Autodesk Inventor part; units mm, degrees
ref_plane "YZ Plane" through (0, 0, 0) normal (1, 0, 0) x (0, 1, 0)
ref_plane "XZ Plane" through (0, 0, 0) normal (0, 1, 0) x (-1, 0, 0)
ref_plane "XY Plane" through (0, 0, 0) normal (0, 0, 1) x (1, 0, 0)
sketch "Sketch1" plane through (0, 0, 0) normal (0, 1, 0) x (-1, 0, 0)
  line L0 (0, -34.641) -> (30, 17.3205) construction
  line L1 (30, 17.3205) -> (-30, 17.3205) construction
  line L2 (-30, 17.3205) -> (0, -34.641) construction
  circle A0 centre (0, 0) radius 34.641 construction
  circle A1 centre (0, -34.641) radius 10
  circle A2 centre (-30, 17.3205) radius 10
  circle A3 centre (30, 17.3205) radius 10
  circle A4 centre (0, 0) radius 20
  line L3 (55, -55) -> (-55, -55)
  line L4 (-55, -55) -> (-55, 55)
  line L5 (-55, 55) -> (55, 55)
  line L6 (55, 55) -> (55, -55)
  circle A5 centre (0, 0) radius 45 construction
  point P0 (0, -55)
  point P1 (55, 0)
  dimension "d0" = 60
  dimension "d1" = 20
  dimension "d2" = 40
  dimension "d3" = 90
  dimension "d4" = 55
extrude "Extrusion1" add sketch "Sketch1" against normal blind 110
sketch "Sketch2" plane through (0, 0, 0) normal (0, 1, 0) x (1, 0, 0)
  circle A0 centre (0, 0) radius 20
  circle A1 centre (-30, -17.3205) radius 10
  circle A2 centre (30, -17.3205) radius 10
  circle A3 centre (0, 34.641) radius 10
  line L0 (-55, 55) -> (55, 55)
  line L1 (-55, -55) -> (-55, 55)
  line L2 (55, -55) -> (-55, -55)
  line L3 (55, 55) -> (55, -55)
  circle A4 centre (0, 34.641) radius 6.25
  circle A5 centre (-30, 17.3205) radius 6.25
  circle A6 centre (-30, -17.3205) radius 6.25
  circle A7 centre (0, -34.641) radius 6.25
  circle A8 centre (30, -17.3205) radius 6.25
  circle A9 centre (30, 17.3205) radius 6.25
  arc A10 (-35.4127, 20.4455) -> (-35.4127, -20.4455) centre (0, 0) ccw
  arc A11 (-24.5873, 14.1955) -> (-24.5873, -14.1955) centre (0, 0) ccw
  arc A12 (0, -40.891) -> (35.4127, -20.4455) centre (0, 0) ccw
  arc A13 (35.4127, 20.4455) -> (0, 40.891) centre (0, 0) ccw
  arc A14 (0, -28.391) -> (24.5873, -14.1955) centre (0, 0) ccw
  arc A15 (24.5873, 14.1955) -> (0, 28.391) centre (0, 0) ccw
  dimension "d7" = 12.5
  dimension "d10" = 360
extrude "Extrusion2" cut sketch "Sketch2" against normal through all contours A11 A6 A10 A1 | A1 A10 A5 A11 | A5 | A14 A8 A12 A2 | A2 A12 A7 A14 | A7 | A3 A15 A4 A13 | A3 A13 A9 A15 | A9 picked at (-34.5635, -9.9186) picked at (25.4365, -24.7224) picked at (8.6846, 33.9839)
sketch "Sketch3" plane through (0, -110, 0) normal (0, -1, 0) x (1, 0, 0)
  line L0 (-55, -55) -> (55, -55)
  line L1 (55, -55) -> (55, 55)
  line L2 (55, 55) -> (-55, 55)
  line L3 (-55, 55) -> (-55, -55)
  arc A0 (7.0121, -27.5115) -> (24.5873, -14.1955) centre (0, 0) ccw
  arc A1 (35.4127, -20.4455) -> (24.5873, -14.1955) centre (30, -17.3205) ccw
  arc A2 (8.4355, -40.0115) -> (35.4127, -20.4455) centre (0, 0) ccw
  arc A3 (7.0121, -27.5115) -> (8.4355, -40.0115) centre (0, -34.641) ccw
  arc A4 (20.3196, 19.8284) -> (0, 28.391) centre (0, 0) ccw
  arc A5 (0, 40.891) -> (0, 28.391) centre (0, 34.641) ccw
  arc A6 (30.4332, 27.3111) -> (0, 40.891) centre (0, 0) ccw
  arc A7 (20.3196, 19.8284) -> (30.4332, 27.3111) centre (30, 17.3205) ccw
  arc A8 (-27.3317, 7.6831) -> (-24.5873, -14.1955) centre (0, 0) ccw
  arc A9 (-35.4127, -20.4455) -> (-24.5873, -14.1955) centre (-30, -17.3205) ccw
  arc A10 (-38.8687, 12.7003) -> (-35.4127, -20.4455) centre (0, 0) ccw
  arc A11 (-27.3317, 7.6831) -> (-38.8687, 12.7003) centre (-30, 17.3205) ccw
  circle A12 centre (0, 0) radius 20
  line L4 (-50, 50) -> (50, 50)
  line L5 (50, 50) -> (50, -50)
  line L6 (50, -50) -> (-50, -50)
  line L7 (-50, -50) -> (-50, 50)
  dimension "d14" = 5
extrude "Extrusion3" cut sketch "Sketch3" against normal blind 100 contours A0 A1 A2 A3 | A4 A5 A6 A7 | A8 A9 A10 A11 | A12 | L4 L5 L6 L7
sketch "Sketch5" plane through (55, 0, -55) normal (0, 0, -1) x (-1, 0, 0)
  circle A0 centre (55, -60) radius 10
  line L0 (110, -110) -> (0, -110)
  line L1 (110, 0) -> (0, 0)
  point P0 (55, 0)
  point P1 (55, -110)
  dimension "d17" = 60
  dimension "d20" = 20
extrude "Extrusion4" cut sketch "Sketch5" against normal through all
sketch "Sketch6" plane through (55, 0, 55) normal (1, 0, 0) x (0, 0, -1)
  circle A0 centre (55, -60) radius 10
  line L0 (110, -110) -> (0, -110)
  line L1 (110, 0) -> (0, 0)
  point P0 (55, 0)
  point P1 (55, -110)
  dimension "d21" = 20
  dimension "d22" = 60
extrude "Extrusion5" cut sketch "Sketch6" against normal up to next
sketch "Sketch7" plane through (-50, -110, 50) normal (1, 0, 0) x (0, 0, -1)
  circle A0 centre (90, 15) radius 5
  line L0 (105, 110) -> (105, 0)
  line L1 (-5, 0) -> (105, 0)
  point P0 (50, 110)
  dimension "d25" = 10
  dimension "d26" = 15
  dimension "d27" = 15
extrude "Extrusion6" cut sketch "Sketch7" against normal through all
properties part number "Case1" material "Steel, Mild, Welded"
CAD build for the part. Positions are in the model's coordinates, mm. A direction names the side the tool comes from. Round coordinates to 2 decimals unless told otherwise and drop trailing zeros. Order: outer loops, then holes, each group sorted by start corner. A loop starts at its lowest first (then second) coordinate and runs counter-clockwise, first axis right, second up. Notation, with made-up numbers: (48.5, -40) -> (102.5, -40) arc R34 cw to (102.5, -3) -> close; hole circle Ø1 at (1, 7.25). An arc over 180 degrees is marked (long way). Write item = value, one per line. Start each with the question number.
(1) Pull direction Y, two halves, no side cores. Call faces 1 (the cylindrical face through (-52, -98, -36)), 2 (the flat face through (-1, -72, 50)), 3 (the flat face through (4, -110, -53)): released by +Y, released by -Y, zero draft, split by the parting line, or undercut.
(2) Cut at B-B, the plane y = -23. List the corners of the cut face in (x, z).
(3) Which spindle directions (+Z, -Z, +X, -X, +Y, -Y) get a long thin tool onto all of the face, cutting with end or side? Do faces 4 (the cylindrical face through (52.54, -69.76, 2.17)), 5 (the flat face through (1, -42, 55)), 6 (the flat face through (-50, -61, -1)), 7 (the cylindrical face through (-6.25, -4.93, 34.5)). Say none if no direction does.
(4) Probe line 1 (Z direction, x = -8.5, y = -38); line 2 (Z direction, x = -30, y = -4.75). List the from-to ranges inside material, lowest first. Write a range as [from, to].
(5) Cut at A-A, the plane x = -12. List the corners of the cut face in (y, z), then the cut area to 3 significant figures.
(6) Pin check, flat tip, straight feed: P1, Ø1, axis at x = 40.5, z = -1, coming from the -Y side. Stop position of the tip, or through.
(7) Cut at D-D, the plane y = -60. List the corners of the cut face in (x, z), then the cut area to 3 significant figures.
(8) Cut at C-C, the plane z = 0. List the corners of the cut face in (x, y).
Model answer:
q1.face_1 = undercut
q1.face_2 = zero draft
q1.face_3 = released by -Y
q2.outline = (-55, -55) -> (55, -55) -> (55, 55) -> (-55, 55) -> close; hole (-50, -50) -> (50, -50) -> (50, 50) -> (-50, 50) -> close
q3.face_4 = +X
q3.face_5 = +Z, +X, -X, +Y, -Y
q3.face_6 = -Y
q3.face_7 = +Y, -Y
q4.line_1 = [-55, -50], [50, 55]
q4.line_2 = [-55, -23.57], [27.32, 55]
q5.outline = (-110, -55) -> (0, -55) -> (0, -16) -> (-10, -16) -> (-10, -50) -> (-110, -50) -> close; (-110, 50) -> (-10, 50) -> (-10, 16) -> (0, 16) -> (0, 55) -> (-110, 55) -> close
q5.area = 1,780 mm2
q6.P1 = -10
q7.outline = (-55, -55) -> (-10, -55) -> (-10, -50) -> (-50, -50) -> (-50, 50) -> (-10, 50) -> (-10, 55) -> (-55, 55) -> close; (10, -55) -> (55, -55) -> (55, -10) -> (50, -10) -> (50, -50) -> (10, -50) -> close; (10, 50) -> (50, 50) -> (50, 10) -> (55, 10) -> (55, 55) -> (10, 55) -> close
q7.area = 1,800 mm2
q8.outline = (-55, -110) -> (-50, -110) -> (-50, -10) -> (-40.89, -10) -> (-40.89, 0) -> (-55, 0) -> close; (-28.39, -10) -> (-20, -10) -> (-20, 0) -> (-28.39, 0) -> close; (20, -10) -> (50, -10) -> (50, -50) -> (55, -50) -> (55, 0) -> (20, 0) -> close; (50, -110) -> (55, -110) -> (55, -70) -> (50, -70) -> close
